from build123d import *

# Parameters (mm, degrees)
SKETCH1_W                      = 38.1
SKETCH1_H                      = 63.5
BOSS_EXTRUDE1_DEPTH            = 3.175
SKETCH2_W                      = 6.35
SKETCH2_H                      = 3.1242
CUT_EXTRUDE1_DEPTH             = 4.175
SKETCH3_W                      = 6.35
SKETCH3_H                      = 3.2258
CUT_FOR_TABS_SERVO_PLATE_DEPTH = 4.175
BASE_EXTENSION_DEPTH           = 3.175
SKETCH5_W                      = 6.35
SKETCH5_H                      = 6.35
SKETCH5_W_2                    = 3.175
TABS_DEPTH                     = 3.175
CUT_FOR_NECK_COVER_TABS_DEPTH  = 4.175
SKETCH7_R                      = 1.7145
CUT_EXTRUDE2_DEPTH             = 4.175


with BuildPart() as part:
    # Sketch1 → Boss-Extrude1 (new body)
    with BuildSketch(Plane(origin=(0, 0, 0), x_dir=(0, 0, -1), z_dir=(1, 0, 0))):
        Rectangle(SKETCH1_W, SKETCH1_H)
    extrude(amount=BOSS_EXTRUDE1_DEPTH)

    # Sketch2 → Cut-Extrude1 (cut, through all)
    with BuildSketch(Plane.ZY):
        with Locations((-10.795, 30.1879)):
            Rectangle(SKETCH2_W, SKETCH2_H)
        with Locations((10.795, 30.1879)):
            Rectangle(SKETCH2_W, SKETCH2_H)
    extrude(amount=-CUT_EXTRUDE1_DEPTH, mode=Mode.SUBTRACT)

    # Sketch3 → cut for tabs servo plate (cut, through all)
    with BuildSketch(Plane.ZY):
        with Locations((-10.795, 14.3891)):
            Rectangle(SKETCH3_W, SKETCH3_H)
        with Locations((10.795, 14.3891)):
            Rectangle(SKETCH3_W, SKETCH3_H)
    extrude(amount=-CUT_FOR_TABS_SERVO_PLATE_DEPTH, mode=Mode.SUBTRACT)

    # Sketch4 → base extension (add)
    with BuildSketch(Plane.ZY):
        Polygon((19.05, -31.75), (63.5, -31.75), (63.5, 3.81), (19.05, 19.295607145), align=None)
    base_extension = extrude(amount=-BASE_EXTENSION_DEPTH)

    # Mirror1: base extension across plane
    add(base_extension.mirror(Plane.XY))

    # Sketch5 → tabs (add)
    with BuildSketch(Plane(origin=(3.175, 0, 0), x_dir=(0, 0, -1), z_dir=(1, 0, 0))):
        with Locations((66.675, -4.445)):
            Rectangle(SKETCH5_W, SKETCH5_H)
        with Locations((66.675, -23.495)):
            Rectangle(SKETCH5_W, SKETCH5_H)
        with Locations((-65.0875, -4.445)):
            Rectangle(SKETCH5_W_2, SKETCH5_H)
        with Locations((-65.0875, -23.495)):
            Rectangle(SKETCH5_W_2, SKETCH5_H)
    extrude(amount=-TABS_DEPTH)

    # Sketch6 → cut for neck cover tabs (cut, through all)
    with BuildSketch(Plane.ZY):
        Polygon((-36.620444722, 9.771864523), (-30.623926297, 11.860947281), (-29.562672256, 8.814715921), (-35.559190682, 6.725633163), align=None)
        Polygon((-48.613481574, 5.593699008), (-47.552227533, 2.547467647), (-53.548745959, 0.45838489), (-54.61, 3.50461625), align=None)
    extrude(amount=-CUT_FOR_NECK_COVER_TABS_DEPTH, mode=Mode.SUBTRACT)

    # Sketch7 → Cut-Extrude2 (cut, through all)
    with BuildSketch(Plane.ZY):
        with Locations((-0.718022777, -25.4)):
            Circle(SKETCH7_R)
    extrude(amount=-CUT_EXTRUDE2_DEPTH, mode=Mode.SUBTRACT)


solid = part.part
The model under review builds one solid part; all positions refer to its coordinate system, in mm. A direction names the side the tool comes from. Round coordinates to 2 decimals unless told otherwise and drop trailing zeros. Write each loop counter-clockwise with the first axis right and the second up, starting at its lowest first coordinate (ties: lowest second). Pieces come first, ordered by that corner, then holes. Notation, with made-up numbers: M 67.5,-3 L 103.5,-3 A4 cw 103.5,1 Z; hole C 16.25,71 d11. An arc over 180 degrees is marked long. Answer as CSV lines item,"result". Start each with the question number.
Q1. Tool access review of faces 1 (the face through (2, -20.32, -67)), 2 (the face through (2, 16.002, -11)), 3 (the face through (2, -7.62, 65)), 4 (the face through (2, -29, 63.5)), 5 (the face through (2, 30, 7.62)): name each direction out of +Z, -Z, +X, -X, +Y, -Y from which nothing blocks a thin tool from reaching the whole face with its end or side.
Q2. Wall thickness on line 1 along Y through (x, z) = (1.85, -10.5); line 2 along Z through (x, y) = (2.75, -11.5); line 3 along Y through (x, z) = (1.5, 0): over which ranges is each line inside the solid? List them lowest first.
Q3. Consider section A-A, the plane y = -25.4. Give the boundary of the cut face in (x, z) (3 decimals).
Q4. Clearance check with flat-ended pins moving along their axes: P1, Ø0.9, axis at x = 1.5, y = 30.5, coming from the +Z side; P2, Ø1, axis at x = 1.5, z = -66.5, coming from the -Y side; P3, Ø1, axis at x = 2, z = -66, coming from the +Y side. State where each tip first meets the part, or that it passes through.
Q5. Consider section B-B, the plane z = 9.5. Give the boundary of the cut face in (x, y) (3 decimals), then the cut area to 3 significant figures.
Q6. Consider section C-C, the plane x = 0.95. State how many separate pieces and enclosed holes the cut face has, then the cut area to 3 significant figures.
Q7. The part is to be moulded in two halves that separate along Z. For faces 6 (the face through (2, 25, 19.05)), 7 (the face through (2, 12.776, 11)), 8 (the face through (2, -14, -63.5)), 9 (the face through (2, 31.75, 0)), say which applies: +Z half, -Z half, draft (parallel to the pull), parting line (faces both ways), or undercut.
Q8. Consider section D-D, the plane y = -15.5. Give the boundary of the cut face in (x, z) (3 decimals).
Result set:
1,face 1,"-Z, +X, -X"
1,face 2,"+X, -X"
1,face 3,"+Z, +X, -X"
1,face 4,"+Z, +X, -X, -Y"
1,face 5,"+X, -X, +Y"
2,line 1,"y = -31.75 to 12.78, 16 to 28.63"
2,line 2,"z = -63.5 to 63.5"
2,line 3,"y = -31.75 to -26.96, -23.84 to 31.75"
3,outline,"M 0,-69.85 L 3.175,-69.85 L 3.175,-2.433 L 0,-2.433 Z; M 0,0.996 L 3.175,0.996 L 3.175,66.675 L 0,66.675 Z"
4,P1,"stops at z = 19.05"
4,P2,"stops at y = -26.67"
4,P3,"stops at y = -1.27"
5,outline,"M 0,-31.75 L 3.175,-31.75 L 3.175,12.776 L 0,12.776 Z; M 0,16.002 L 3.175,16.002 L 3.175,28.626 L 0,28.626 Z"
5,area,"181 mm²"
6,separate pieces,"1"
6,enclosed holes,"5"
6,area,"6,260 mm²"
7,face 6,"+Z half"
7,face 7,"undercut"
7,face 8,"-Z half"
7,face 9,"draft"
8,outline,"M 0,-63.5 L 3.175,-63.5 L 3.175,63.5 L 0,63.5 Z"
